```python
from build123d import *

# Parameters (mm, degrees)
SKETCH1_R           = 8.5
SKETCH1_R_2         = 1.5
BOSS_EXTRUDE1_DEPTH = 6.5
BOSS_EXTRUDE3_DEPTH = 14.82
BOSS_EXTRUDE4_START = -3
SKETCH4_R           = 1.5
BOSS_EXTRUDE4_DEPTH = 3


with BuildPart() as part:
    # Sketch1 → Boss-Extrude1 (new body)
    with BuildSketch(Plane(origin=(0, 0, 0), x_dir=(1, 0, 0), z_dir=(0, 1, 0))):
        with BuildLine():
            Line((-15.5, -31), (-15.5, -42.246301613))
            ThreePointArc((-15.5, -42.246301613), (-31.819805153, 31.819805153), (42.246301613, 15.5))
            Line((42.246301613, 15.5), (31, 15.5))
            ThreePointArc((31, 15.5), (23.928932188, 12.571067812), (21, 5.5))
            Line((21, 5.5), (21, -11))
            ThreePointArc((21, -11), (18.071067812, -18.071067812), (11, -21))
            Line((11, -21), (-5.5, -21))
            ThreePointArc((-5.5, -21), (-12.571067812, -23.928932188), (-15.5, -31))
        make_face()
        with Locations(Location((0, 0, 0), (0, 0, 90))):
            Circle(SKETCH1_R, mode=Mode.SUBTRACT)
        with Locations(Location((-7.75, 13.423393759, 0), (0, 0, 90))):
            Circle(SKETCH1_R_2, mode=Mode.SUBTRACT)
        with Locations(Location((7.75, 13.423393759, 0), (0, 0, 90))):
            Circle(SKETCH1_R_2, mode=Mode.SUBTRACT)
        with Locations(Location((15.5, 0, 0), (0, 0, 90))):
            Circle(SKETCH1_R_2, mode=Mode.SUBTRACT)
        with Locations(Location((-15.5, 0, 0), (0, 0, 90))):
            Circle(SKETCH1_R_2, mode=Mode.SUBTRACT)
        with Locations(Location((-7.75, -13.423393759, 0), (0, 0, 90))):
            Circle(SKETCH1_R_2, mode=Mode.SUBTRACT)
        with Locations(Location((7.75, -13.423393759, 0), (0, 0, 90))):
            Circle(SKETCH1_R_2, mode=Mode.SUBTRACT)
    extrude(amount=BOSS_EXTRUDE1_DEPTH)

    # Sketch3 → Boss-Extrude3 (add)
    with BuildSketch(Plane(origin=(0, 6.5, 0), x_dir=(1, 0, 0), z_dir=(0, 1, 0))):
        with BuildLine():
            Line((42.246301613, 15.5), (39.035240489, 15.5))
            ThreePointArc((39.035240489, 15.5), (-29.69848481, 29.69848481), (-15.5, -39.035240489))
            Line((-15.5, -39.035240489), (-15.5, -42.246301613))
            ThreePointArc((-15.5, -42.246301613), (-31.819805153, 31.819805153), (42.246301613, 15.5))
        make_face()
    extrude(amount=BOSS_EXTRUDE3_DEPTH)

    # Sketch4 → Boss-Extrude4 (add)
    with BuildSketch(Plane(origin=(0, 21.32, 0), x_dir=(1, 0, 0), z_dir=(0, 1, 0)).offset(BOSS_EXTRUDE4_START)):
        with BuildLine():
            Line((42.246301613, 15.5), (43.205902375, 15.5))
            ThreePointArc((43.205902375, 15.5), (45.710154078, 16.848115196), (45.96372593, 19.680851064))
            ThreePointArc((45.96372593, 19.680851064), (-35.355339059, 35.355339059), (-19.680851064, -45.96372593))
            ThreePointArc((-19.680851064, -45.96372593), (-16.848115196, -45.710154078), (-15.5, -43.205902375))
            Line((-15.5, -43.205902375), (-15.5, -42.246301613))
            ThreePointArc((-15.5, -42.246301613), (-31.819805153, 31.819805153), (42.246301613, 15.5))
        make_face()
        with Locations(Location((-33.587572106, 33.587572106, 0), (0, 0, 270))):
            Circle(SKETCH4_R, mode=Mode.SUBTRACT)
        with Locations(Location((-33.587572106, -33.587572106, 0), (0, 0, 270))):
            Circle(SKETCH4_R, mode=Mode.SUBTRACT)
        with Locations(Location((33.587572106, 33.587572106, 0), (0, 0, 270))):
            Circle(SKETCH4_R, mode=Mode.SUBTRACT)
    extrude(amount=BOSS_EXTRUDE4_DEPTH)


solid = part.part
```
Verification items for the finished model (mm, model axes). A direction names the side the tool comes from. Give positions to 0.01 mm unless a question says otherwise; leave off trailing zeros. Order: outer loops, then holes, each group sorted by start corner. A loop starts at its lowest first (then second) coordinate and runs counter-clockwise, first axis right, second up. Notation, with made-up numbers: (5.25, 63) - (24.25, 63) arc R31 ccw to (24.25, 102) - close; hole circle Ø5 at (3, 56.25). An arc over 180 degrees is marked (long way). Answer as CSV lines item,"result". Start each with the question number.
Item 1: Section check C-C, the plane x = 0. Record the boundary of the cut face in (y, z), plus the area to 3 significant figures.
Item 2: Section check B-B, the plane y = 1.75. Record the boundary of the cut face in (x, z).
Item 3: Access from +Z, -Z, +X, -X, +Y, -Y to the whole of each face (thin tool, end or side, straight path). Record for faces 1 (the face through (38, 6, -15.5)), 2 (the face through (-32.7, 9.032, -30.914)), 3 (the face through (35.075, 19.799, -33.783)), 4 (the face through (-28.865, 13.806, -30.509)).
Item 4: Section check A-A, the plane z = 0. Record the boundary of the cut face in (x, y).
Item 5: Mould release check, pull along X, two halves, no side actions. Record for faces 5 (the face through (-15.5, 6, 39)), 6 (the face through (-35.052, 19.799, -33.913)), 7 (the face through (3, 3, 21)): released by +X, released by -X, zero draft, split by the parting line, or undercut.
Item 6: Section check D-D, the plane x = -18.5. Record the boundary of the cut face in (y, z), plus the area to 3 significant figures.
Item 7: Material ranges on L1, parallel to Z at x = 7.75, y = 2; L2, parallel to Z at x = -7.75, y = 3.5; L3, parallel to Y at x = -13, z = -22, recorded low to high.
Item 8: Gauge pin test, flat ends, axial feed: pin 1 (10 mm diameter, centred on y = 5.5, z = 26, fed in from -X); pin 2 (5 mm diameter, centred on x = -33.59, z = -33.59, fed in from +Y); pin 3 (5 mm diameter, centred on x = -7.75, z = -13.42, fed in from +Y); pin 4 (10 mm diameter, centred on x = 0, z = 0, fed in from +Y). Record the tip position at first contact, or that the pin passes through.
Filled in:
1,outline,"(0, -45) - (18.32, -45) - (18.32, -50) - (21.32, -50) - (21.32, -42) - (6.5, -42) - (6.5, -8.5) - (0, -8.5) - close; (0, 8.5) - (6.5, 8.5) - (6.5, 21) - (0, 21) - close"
1,area,"378 mm^2"
2,outline,"(-15.5, 31) - (-15.5, 42.25) arc R45 ccw (long way) to (42.25, -15.5) - (31, -15.5) arc R10 cw to (21, -5.5) - (21, 11) arc R10 ccw to (11, 21) - (-5.5, 21) arc R10 cw to start; hole circle Ø3 at (-15.5, 0); hole circle Ø3 at (-7.75, -13.42); hole circle Ø3 at (-7.75, 13.42); hole circle Ø17 at (0, 0); hole circle Ø3 at (7.75, -13.42); hole circle Ø3 at (7.75, 13.42); hole circle Ø3 at (15.5, 0)"
3,face 1,"+Z, +X, +Y, -Y"
3,face 2,"-Y"
3,face 3,"+Y, -Y"
3,face 4,"+Y"
4,outline,"(-50, 18.32) - (-45, 18.32) - (-45, 0) - (-17, 0) - (-17, 6.5) - (-42, 6.5) - (-42, 21.32) - (-50, 21.32) - close; (-14, 0) - (-8.5, 0) - (-8.5, 6.5) - (-14, 6.5) - close; (8.5, 0) - (14, 0) - (14, 6.5) - (8.5, 6.5) - close; (17, 0) - (21, 0) - (21, 6.5) - (17, 6.5) - close"
5,face 5,"released by +X"
5,face 6,"undercut"
5,face 7,"zero draft"
6,outline,"(0, -41.02) - (18.32, -41.02) - (18.32, -46.45) - (21.32, -46.45) - (21.32, -37.71) - (6.5, -37.71) - (6.5, 37.71) - (21.32, 37.71) - (21.32, 46.21) - (18.32, 46.21) - (18.32, 41.02) - (0, 41.02) - close"
6,area,"663 mm^2"
7,L1,"-44.33 to -14.92, -11.92 to -3.49, 3.49 to 11.92, 14.92 to 21"
7,L2,"-44.33 to -14.92, -11.92 to -3.49, 3.49 to 11.92, 14.92 to 21.26"
7,L3,"0 to 6.5"
8,pin 1,"x = -39.8"
8,pin 2,"y = 21.32"
8,pin 3,"y = 6.5"
8,pin 4,"through"
